Here's the drawing with two shaded views (mm, measured from the low corner). I have some questions. A direction names the side the tool comes from. Give positions to 0.01 mm unless a question says otherwise; leave off trailing zeros. Write each loop counter-clockwise with the first axis right and the second up, starting at its lowest first coordinate (ties: lowest second). Pieces come first, ordered by that corner, then holes. Notation, with made-up numbers: (14, -19) - (23, -19) arc R18 ccw to (23, 3) - close; hole circle Ø1 at (-17.75, -32). An arc over 180 degrees is marked (long way). Answer as a JSON object with one key per item and string values. Group by question number.
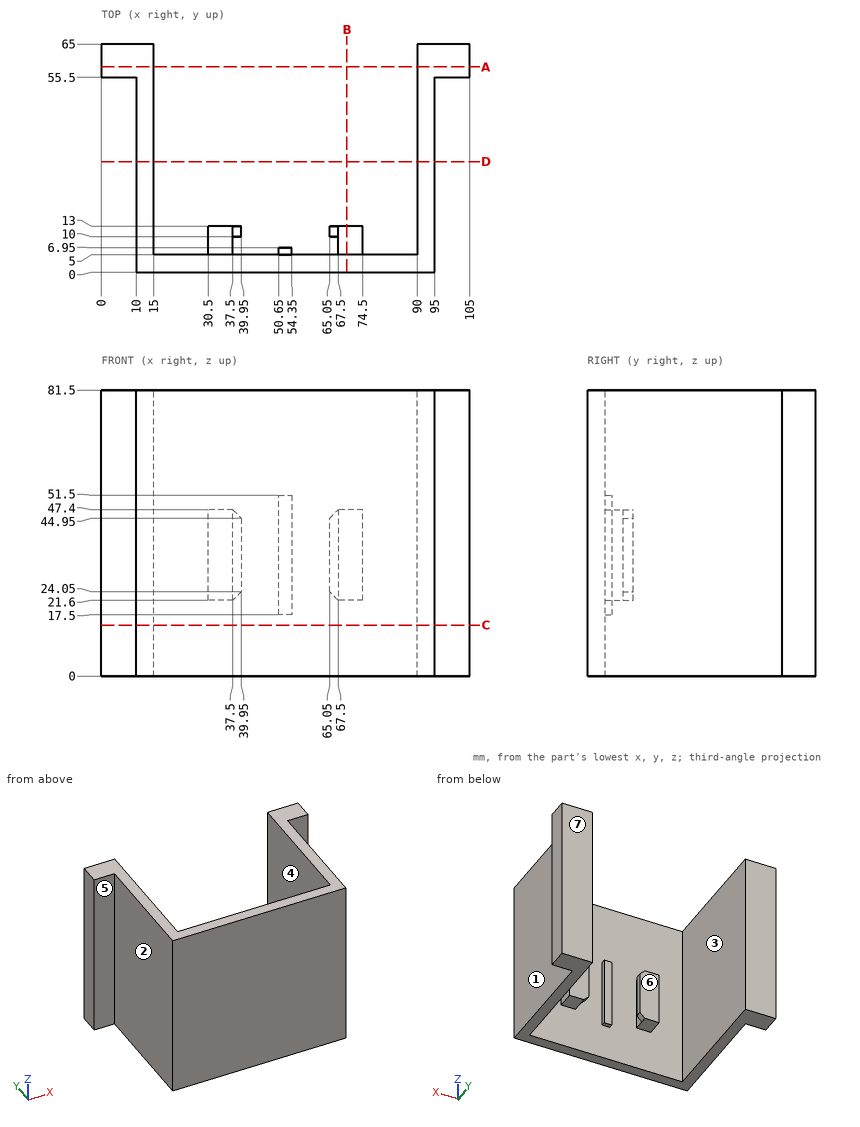
(1) Will these pins go through, and if not, where does the flat tip stop? P1, Ø10.5, axis at x = 67.5, z = 33, coming from the +Y side; P2, Ø8, axis at y = 35, z = 62, coming from the -X side; P3, Ø3, axis at y = 10.5, z = 28, coming from the +X side.
(2) I want a section at A-A, the plane y = 58.5. Please give me the cut outline in (x, z), and give its area (4 significant figures).
(3) If we mould it in two halves opening along X, with no side actions, what happens to the marked faces 1, 2, 3 and 4? For each: +X half, -X half, draft (parallel to the pull), parting line (faces both ways), or undercut.
(4) I want a section at D-D, the plane y = 31.5. Please give me the cut outline in (x, z).
(5) For the marked faces 5, 6 and 7, which set-ups out of +Z, -Z, +X, -X, +Y, -Y let a thin tool reach every point of the face, with its end or its side?
(6) I want a section at C-C, the plane z = 14.5. Please give me the cut outline in (x, y).
(7) I need wall thicknesses on L1, parallel to X at y = 58.5, z = 9.5; L2, parallel to X at y = 27.5, z = 5.5; L3, parallel to Y at x = 38, z = 36. Which ranges of each line are inside material? Lowest first, please.
(8) I want a section at B-B, the plane x = 70. Please give me the cut outline in (y, z), and give its area (3 significant figures).
Entries:
{
 "1": {"P1": "y = 13", "P2": "x = 10", "P3": "x = 95"},
 "2": {"outline": "(0, 0) - (15, 0) - (15, 81.5) - (0, 81.5) - close; (90, 0) - (105, 0) - (105, 81.5) - (90, 81.5) - close", "area": "2,445 mm^2"},
 "3": {"face 1": "+X half", "face 2": "-X half", "face 3": "undercut", "face 4": "undercut"},
 "4": {"outline": "(10, 0) - (15, 0) - (15, 81.5) - (10, 81.5) - close; (90, 0) - (95, 0) - (95, 81.5) - (90, 81.5) - close"},
 "5": {"face 5": "+Z, -Z, -X, -Y", "face 6": "+Z, -Z, +Y", "face 7": "+Z, -Z, +X, -X, +Y"},
 "6": {"outline": "(0, 55.5) - (10, 55.5) - (10, 0) - (95, 0) - (95, 55.5) - (105, 55.5) - (105, 65) - (90, 65) - (90, 5) - (15, 5) - (15, 65) - (0, 65) - close"},
 "7": {"L1": "0 to 15, 90 to 105", "L2": "10 to 15, 90 to 95", "L3": "0 to 5, 10 to 13"},
 "8": {"outline": "(0, 0) - (5, 0) - (5, 21.6) - (13, 21.6) - (13, 47.4) - (5, 47.4) - (5, 81.5) - (0, 81.5) - close", "area": "614 mm^2"}
}
